For this review, take the finished solid that the model builds, in its own axes (mm). A direction names the side the tool comes from. Coordinates: 2 decimals unless noted, no trailing zeros. Loops run counter-clockwise (first coordinate to the right, second up) from the corner with the lowest first, then second, coordinate; pieces in that order, holes last.
1. Take a section at C-C, the plane y = 19.5. State the section outline as (x, z) points.
2. Mouldability with a two-part tool opening along X and no side actions: class faces 1 (the face through (-60.67, -14.47, 15.07)), 2 (the face through (-27.706, -16.591, 15.07)), 3 (the face through (-45, 23, 15)), 4 (the face through (57, -25, 10)) as pulls with the +X half, pulls with the -X half, needs draft (parallel to the pull), parting line crosses it, or undercut.
3. Machinability: for faces 5 (the face through (-33, 11, 10)), 6 (the face through (0, 10, 10)), 7 (the face through (48.335, -24.986, 3.216)), which of the approach directions +Z, -Z, +X, -X, +Y, -Y give a long, thin tool a straight path to every point of the face, cutting with its end or side? Answer none if there is none.
4. Clearance check with flat-ended pins moving along their axes: P1, Ø3, axis at y = 1, z = 14.5, coming from the -X side; P2, Ø10, axis at x = -8, z = 15, coming from the -Y side; P3, Ø4, axis at y = -20, z = 6.5, coming from the -X side. State where each tip first meets the part, or that it passes through.
5. Take a section at D-D, the plane y = 2.5. State the section outline as (x, z) points, then the cut area to 3 significant figures.
6. To check wall thickness, follow probe 1 along Z at (x, y) = (47, -24.75) (3 decimals); probe 2 along Y at (x, z) = (-41.5, 17); probe 3 along Y at (x, z) = (41, 2). State the ranges of each line that lie inside material, in increasing order.
7. Take a section at B-B, the plane y = 12. State the section outline as (x, z) points.
8. Take a section at A-A, the plane x = 24. State the section outline as (y, z) points, then the cut area to 3 significant figures.
```python
from build123d import *

# Parameters (mm, degrees)
SKETCH_W     = 40
SKETCH_H     = 20
PAD_DEPTH    = 20
SKETCH001_W  = 48
SKETCH001_H  = 20
PAD001_DEPTH = 2
SKETCH002_R  = 1.4
PAD002_DEPTH = 2
SKETCH003_R  = 3.5
PAD003_DEPTH = 2
PAD004_DEPTH = 10
CHAMFER_SIZE = 9.5


with BuildPart() as part:
    # Sketch → Pad (new body)
    with BuildSketch(Plane.XY):
        Rectangle(SKETCH_W, SKETCH_H)
    extrude(amount=PAD_DEPTH)

    # Sketch001 (on Face2 of Pad) → Pad001 (join)
    with BuildSketch(Plane.YZ.offset(20)):
        with Locations((0, 10)):
            Rectangle(SKETCH001_W, SKETCH001_H)
    extrude(amount=PAD001_DEPTH)

    # Sketch002 (on Face2 of Pad001) → Pad002 (join)
    with BuildSketch(Plane.XZ.offset(24)):
        with BuildLine():
            Line((20, 20), (47, 20))
            ThreePointArc((47, 0), (57, 10), (47, 20))
            Line((20, 0), (47, 0))
            Line((20, 20), (20, 0))
        make_face()
        with Locations((47, 10)):
            Circle(SKETCH002_R, mode=Mode.SUBTRACT)
        with Locations((47, 17.205)):
            Circle(SKETCH002_R, mode=Mode.SUBTRACT)
        with Locations((53.934549, 10)):
            Circle(SKETCH002_R, mode=Mode.SUBTRACT)
        with Locations((47, 2.795)):
            Circle(SKETCH002_R, mode=Mode.SUBTRACT)
        with Locations((40.065451, 10)):
            Circle(SKETCH002_R, mode=Mode.SUBTRACT)
    extrude(amount=PAD002_DEPTH)

    # Sketch003 (on Face3 of Pad002) → Pad003 (join)
    with BuildSketch(Plane(origin=(0, 24, 0), x_dir=(-1, 0, 0), z_dir=(0, 1, 0))):
        with BuildLine():
            Line((-20, 20), (-47, 20))
            ThreePointArc((-47, 20), (-57, 10), (-47, 0))
            Line((-20, 0), (-47, 0))
            Line((-20, 20), (-20, 0))
        make_face()
        with Locations((-47, 10)):
            Circle(SKETCH003_R, mode=Mode.SUBTRACT)
    extrude(amount=PAD003_DEPTH)

    # Sketch004 (on Face5 of Pad003) → Pad004 (join)
    with BuildSketch(Plane.XY.offset(20)):
        Polygon((-20, 10), (-35.198684, 23), (-55.198684, 23), (-66, 6.167544), (-58, 6.167544), (-52.33225, 15), (-38.326285, 15), (-28, 6.167544), (-28, -6.167544), (-38.326285, -15), (-52.33225, -15), (-58, -6.167544), (-66, -6.167544), (-55.198684, -23), (-35.198684, -23), (-20, -10), align=None)
    extrude(amount=-PAD004_DEPTH)

    # Chamfer
    chamfer_edges = [part.edges().sort_by_distance(p)[0] for p in [
        (-20, 0, 0),
    ]]
    chamfer(chamfer_edges, length=CHAMFER_SIZE)


solid = part.part
```
Results list:
1. outline: (-57.44, 10) - (-31.11, 10) - (-31.11, 20) - (-57.44, 20) - close; (20, 0) - (22, 0) - (22, 20) - (20, 20) - close
2. face 1: pulls with the -X half
2. face 2: undercut
2. face 3: needs draft
2. face 4: pulls with the +X half
3. face 5: -Z, -X, +Y, -Y
3. face 6: +Z, -Z, +Y
3. face 7: -Y
4. P1: stops at x = -28
4. P2: stops at y = -10
4. P3: stops at x = 20
5. outline: (-28, 10) - (-20, 10) - (-20, 9.5) - (-10.5, 0) - (22, 0) - (22, 20) - (-28, 20) - close
5. area: 875 mm2
6. probe 1: z = 0 to 1.395, 4.195 to 8.6, 11.4 to 15.805, 18.605 to 20
6. probe 2: y = -23 to -15, 15 to 23
6. probe 3: y = -26 to -24, 24 to 26
7. outline: (-62.26, 10) - (-54.26, 10) - (-54.26, 20) - (-62.26, 20) - close; (-34.82, 10) - (-22.34, 10) - (-22.34, 20) - (-34.82, 20) - close; (20, 0) - (22, 0) - (22, 20) - (20, 20) - close
8. outline: (-26, 0) - (-24, 0) - (-24, 20) - (-26, 20) - close; (24, 0) - (26, 0) - (26, 20) - (24, 20) - close
8. area: 80.0 mm2
